The drawing under review shows one solid part. Ordinate dimensions are in mm from its lowest x, y, z. A direction names the side the tool comes from. Give positions to 0.01 mm unless a question says otherwise; leave off trailing zeros. Order: outer loops, then holes, each group sorted by start corner. A loop starts at its lowest first (then second) coordinate and runs counter-clockwise, first axis right, second up. Notation, with made-up numbers: (27.5, 79) - (57.5, 79) arc R20 ccw to (57.5, 116) - close; hole circle Ø5 at (30.5, -16). An arc over 180 degrees is marked (long way). Write item = value, one per line. Start each with the question number.
1. Mouldability with a two-part tool opening along X and no side actions: class the marked faces 1, 2 and 3 as pulls with the +X half, pulls with the -X half, needs draft (parallel to the pull), parting line crosses it, or undercut.
2. Machinability: for the marked faces 4 and 5, which of the approach directions +Z, -Z, +X, -X, +Y, -Y give a long, thin tool a straight path to every point of the face, cutting with its end or side? Answer none if there is none.
3. We need section B-B, the plane z = 3.5. Give the boundary of the cut face in (x, y).
4. We need section A-A, the plane z = 8.75. Give the boundary of the cut face in (x, y).
5. For P1, Ø1, axis at x = 0.5, y = 3.5, coming from the -Z side; P2, Ø1.5, axis at x = 2.5, z = 6.5, coming from the +Y side; P3, Ø2, axis at y = 3.5, z = 7.5, coming from the +X side, all flat-tipped, find the tip position at first contact; note any pin that passes through.
6. Wall thickness on probe 1 along X at (y, z) = (2, 7) (1 decimal); probe 2 along Z at (x, y) = (1.15, 3.7); probe 3 along Y at (x, z) = (2.2, 11.75): over which ranges is each line inside the solid? List them lowest first.
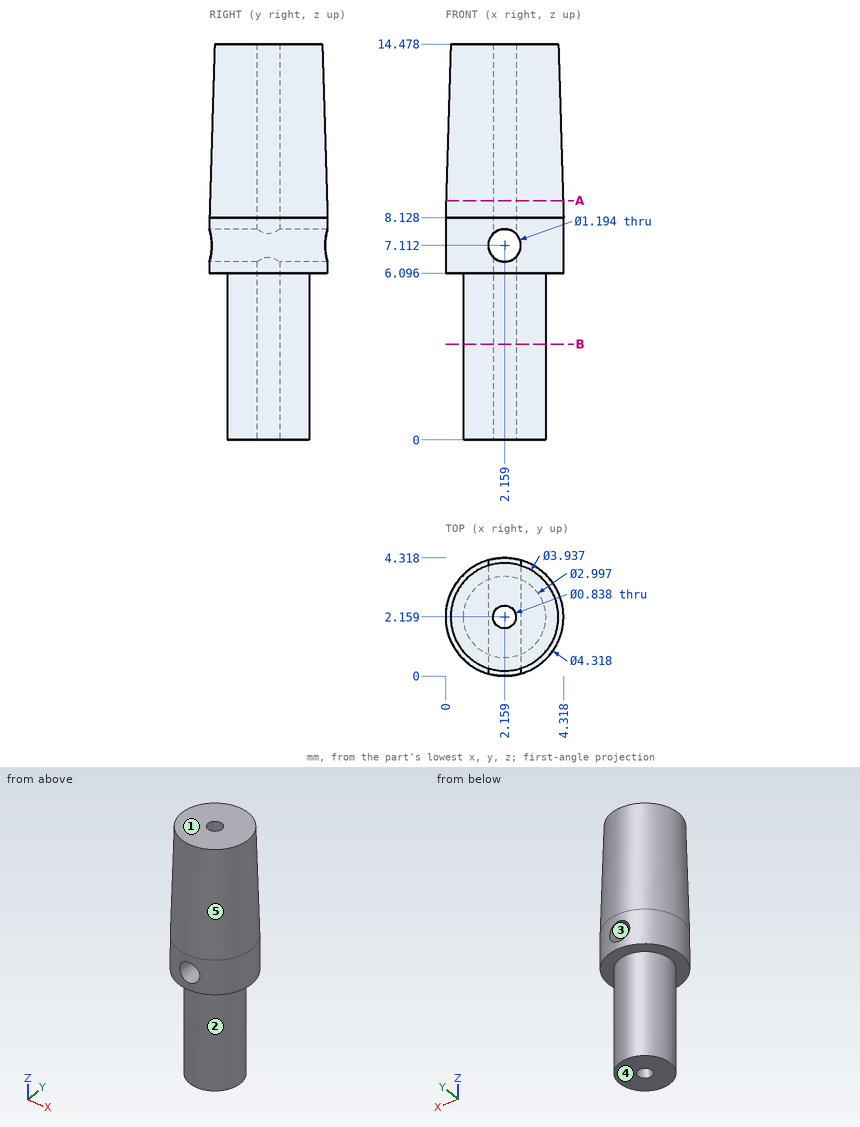
Model answer:
q1.face_1 = needs draft
q1.face_2 = parting line crosses it
q1.face_3 = undercut
q2.face_4 = -Z, +X, -X, +Y, -Y
q2.face_5 = +Z
q3.outline = circle Ø3 at (2.16, 2.16); hole circle Ø0.84 at (2.16, 2.16)
q4.outline = circle Ø4.28 at (2.16, 2.16); hole circle Ø0.84 at (2.16, 2.16)
q5.P1 = 6.1
q5.P2 = 4.32
q5.P3 = 4.29
q6.probe_1 = 0 to 1.6, 2.7 to 4.3
q6.probe_2 = 6.1 to 14.48
q6.probe_3 = 0.11 to 1.74, 2.58 to 4.21
